Part model, mm, in its own coordinate system. Face numbers are marked on the shaded views. A direction names the side the tool comes from. Round coordinates to 2 decimals unless told otherwise and drop trailing zeros. Write each loop counter-clockwise with the first axis right and the second up, starting at its lowest first coordinate (ties: lowest second). Pieces come first, ordered by that corner, then holes. Notation, with made-up numbers: M 81.25,60 L 114.25,60 A10 cw 114.25,69 Z; hole C 58,-32.5 d4. An arc over 180 degrees is marked long. Use a Markdown table: item, result. Add a question column.
1) Slice it at B-B on y = -41. Write the cut outline in (x, z), plus the area to 3 significant figures.
2) Slice it at A-A on x = 7. Write the cut outline in (y, z), plus the area to 3 significant figures.
3) Wall check: probe 1 along X at (y, z) = (-40.5, 58.5); probe 2 along X at (y, z) = (-18.5, -26); probe 3 along Z at (x, y) = (17.5, -10). Give the ranges that are in metal, low to high.
4) Drop flat-ended pins along their axis: P1, Ø6, axis at y = -22, z = -19.5, coming from the +X side; P2, Ø0.7, axis at y = -18.7, z = -9.91, coming from the -X side; P3, Ø1.6, axis at y = -22.26, z = 66.31, coming from the -X side; P4, Ø2, axis at y = 2.5, z = -10.5, coming from the -X side. Give the stop position or say it passes through.
5) Which spindle directions (+Z, -Z, +X, -X, +Y, -Y) get a long thin tool onto all of the face, cutting with end or side? Do the marked faces 1, 2, 3 and 4. Say none if no direction does.
```python
from build123d import *

# Parameters (mm, degrees)
SKETCH_1_W           = 20
SKETCH_1_H           = 40
EXTRUDE_1_DEPTH      = 40
SKETCH_2_R           = 0.6
CUT_EXTRUDE_1_DEPTH  = 5
EXTRUDE_3_DEPTH      = 5
EXTRUDE_3_DEPTH_BACK = 45
SKETCH_3_R           = 3
SKETCH_4_R           = 1
CUT_EXTRUDE_2_DEPTH  = 5
EXTRUDE_START        = -3
SKETCH_5_R           = 1
EXTRUDE_4_DEPTH      = 3


with BuildPart() as part:
    # ｽｹｯﾁ1 → ﾎﾞｽ - 押し出し1 (new body)
    with BuildSketch(Plane(origin=(0, 0, 0), x_dir=(0, 0, -1), z_dir=(1, 0, 0))):
        with Locations((18.409001804, -0.200935369)):
            Rectangle(SKETCH_1_W, SKETCH_1_H)
    extrude(amount=EXTRUDE_1_DEPTH)

    # ｽｹｯﾁ2 → ｶｯﾄ - 押し出し1 (cut)
    with BuildSketch(Plane(origin=(40, 0, 0), x_dir=(0, 0, -1), z_dir=(1, 0, 0))):
        with Locations((26.909001804, -18.700935369)):
            Circle(SKETCH_2_R)
        with Locations((26.909001804, -3.700935369)):
            Circle(SKETCH_2_R)
        with Locations(Location((9.909001804, -3.700935369, 0), (0, 0, 180))):
            Circle(SKETCH_2_R)
        with Locations(Location((9.909001804, -18.700935369, 0), (0, 0, 180))):
            Circle(SKETCH_2_R)
    extrude(amount=-CUT_EXTRUDE_1_DEPTH, mode=Mode.SUBTRACT)

    # ｽｹｯﾁ3 → ﾎﾞｽ - 押し出し3 (add, two sides: drawn at the far end of the back side and taken through both)
    with BuildSketch(Plane(origin=(40, 0, 0), x_dir=(0, 0, -1), z_dir=(1, 0, 0)).offset(-EXTRUDE_3_DEPTH_BACK)):
        with Locations((18.409001804, 11.299064631)):
            Circle(SKETCH_3_R)
    extrude(amount=EXTRUDE_3_DEPTH + EXTRUDE_3_DEPTH_BACK)

    # ｽｹｯﾁ4 → ｶｯﾄ - 押し出し2 (cut)
    with BuildSketch(Plane.ZY):
        with Locations((-11.409001804, -13.700935369)):
            Circle(SKETCH_4_R)
        with Locations((-25.409001804, -13.700935369)):
            Circle(SKETCH_4_R)
        with Locations(Location((-26.409001804, 2.299064631, 0), (0, 0, 180))):
            Circle(SKETCH_4_R)
        with Locations((-10.409001804, 2.299064631)):
            Circle(SKETCH_4_R)
        with Locations((-11.409001804, -10.700935369)):
            Circle(SKETCH_4_R)
        with Locations(Location((-25.409001804, -10.700935369, 0), (0, 0, 180))):
            Circle(SKETCH_4_R)
        with Locations((-18.409001804, -17.200935369)):
            Circle(SKETCH_4_R)
    extrude(amount=-CUT_EXTRUDE_2_DEPTH, mode=Mode.SUBTRACT)

    # ｽｹｯﾁ5 → ﾎﾞｽ - 押し出し4 (add)
    with BuildSketch(Plane(origin=(0, 0, 0), x_dir=(0, 0, -1), z_dir=(1, 0, 0)).offset(EXTRUDE_START)):
        Polygon((34.742298306, -2.699182148), (-56.038607458, -2.699182148), (-73.963087357, -17.71777437), (-73.963087357, -73.523937735), (-56.038607458, -88.542529958), (34.742298306, -88.542529958), align=None)
        with Locations(Location((11.409001804, -10.700935369, 0), (0, 0, 180))):
            Circle(SKETCH_5_R, mode=Mode.SUBTRACT)
        with Locations(Location((11.409001804, -13.700935369, 0), (0, 0, 180))):
            Circle(SKETCH_5_R, mode=Mode.SUBTRACT)
        with Locations(Location((18.409001804, -17.200935369, 0), (0, 0, 180))):
            Circle(SKETCH_5_R, mode=Mode.SUBTRACT)
        with Locations((25.409001804, -10.700935369)):
            Circle(SKETCH_5_R, mode=Mode.SUBTRACT)
        with Locations(Location((25.409001804, -13.700935369, 0), (0, 0, 180))):
            Circle(SKETCH_5_R, mode=Mode.SUBTRACT)
        with Locations((-66.307722518, -36.25601617)):
            Circle(SKETCH_5_R, mode=Mode.SUBTRACT)
        with Locations((-63.307722518, -36.25601617)):
            Circle(SKETCH_5_R, mode=Mode.SUBTRACT)
        with Locations((-59.807722518, -29.25601617)):
            Circle(SKETCH_5_R, mode=Mode.SUBTRACT)
        with Locations((-66.307722518, -22.25601617)):
            Circle(SKETCH_5_R, mode=Mode.SUBTRACT)
        with Locations((-63.307722518, -22.25601617)):
            Circle(SKETCH_5_R, mode=Mode.SUBTRACT)
        with Locations(Location((25.409001804, -77.540776736, 0), (0, 0, 180))):
            Circle(SKETCH_5_R, mode=Mode.SUBTRACT)
        with Locations(Location((25.409001804, -80.540776736, 0), (0, 0, 180))):
            Circle(SKETCH_5_R, mode=Mode.SUBTRACT)
        with Locations(Location((18.409001804, -74.040776736, 0), (0, 0, 180))):
            Circle(SKETCH_5_R, mode=Mode.SUBTRACT)
        with Locations(Location((11.409001804, -77.540776736, 0), (0, 0, 180))):
            Circle(SKETCH_5_R, mode=Mode.SUBTRACT)
        with Locations(Location((11.409001804, -80.540776736, 0), (0, 0, 180))):
            Circle(SKETCH_5_R, mode=Mode.SUBTRACT)
        with Locations(Location((-63.307722518, -68.985695936, 0), (0, 0, 180))):
            Circle(SKETCH_5_R, mode=Mode.SUBTRACT)
        with Locations(Location((-66.307722518, -68.985695936, 0), (0, 0, 180))):
            Circle(SKETCH_5_R, mode=Mode.SUBTRACT)
        with Locations(Location((-59.807722518, -61.985695936, 0), (0, 0, 180))):
            Circle(SKETCH_5_R, mode=Mode.SUBTRACT)
        with Locations(Location((-63.307722518, -54.985695936, 0), (0, 0, 180))):
            Circle(SKETCH_5_R, mode=Mode.SUBTRACT)
        with Locations(Location((-66.307722518, -54.985695936, 0), (0, 0, 180))):
            Circle(SKETCH_5_R, mode=Mode.SUBTRACT)
    extrude(amount=EXTRUDE_4_DEPTH)


solid = part.part
```
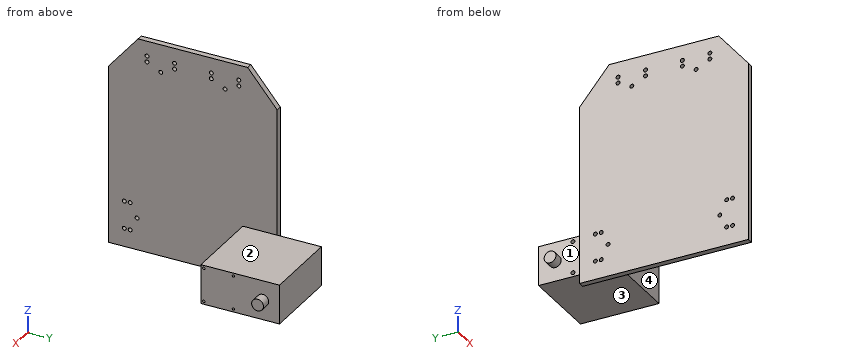
Entries:
| question | item | result |
|---|---|---|
| 1 | outline | M -3,-34.74 L 0,-34.74 L 0,73.96 L -3,73.96 Z |
| 1 | area | 326 mm^2 |
| 2 | outline | M -20.2,-28.41 L 19.8,-28.41 L 19.8,-8.41 L -20.2,-8.41 Z |
| 2 | area | 800 mm^2 |
| 3 | probe 1 | x = -3 to 0 |
| 3 | probe 2 | x = -3 to 40 |
| 3 | probe 3 | z = -28.41 to -8.41 |
| 4 | P1 | stops at x = 40 |
| 4 | P2 | stops at x = -3 |
| 4 | P3 | passes through |
| 4 | P4 | stops at x = 0 |
| 5 | face 1 | -X |
| 5 | face 2 | +Z, +X, +Y, -Y |
| 5 | face 3 | -Z, +X, +Y, -Y |
| 5 | face 4 | +Z, -Z, +X, -Y |
